Design review of the part shown in the three views and the two pictorial views. Dimensions are in mm from the part's minimum x, y and z. A direction names the side the tool comes from. Coordinates: 2 decimals unless noted, no trailing zeros. Loops run counter-clockwise (first coordinate to the right, second up) from the corner with the lowest first, then second, coordinate; pieces in that order, holes last.
Q1. Wall thickness on probe 1 along Z at (x, y) = (78.5, 21) (1 decimal); probe 2 along Y at (x, z) = (34, 14.25) (1 decimal); probe 3 along Z at (x, y) = (114, 1): over which ranges is each line inside the solid? List them lowest first.
Q2. Add section D-D on x = 115.5. Give the boundary of the cut face in (y, z) (1 decimal), and give its area (3 significant figures).
Q3. For P1, Ø7.5, axis at x = 114.3, z = 12.7, coming from the +Y side (3 decimals), flat-tipped, find the tip position at first contact; note if it passes through.
Q4. Machinability: for the marked faces 1 and 2, which of the approach directions +Z, -Z, +X, -X, +Y, -Y give a long, thin tool a straight path to every point of the face, cutting with its end or side? Answer none if there is none.
Q5. Add section B-B on x = 53. Give the boundary of the cut face in (y, z) (1 decimal).
Q6. Draft analysis for pull direction Z (two halves, no side actions). For the marked faces 3, 4, 5 and 6, state which applies: released by +Z, released by -Z, zero draft, split by the parting line, or undercut.
Q7. Add section C-C on y = 14.5. Give the boundary of the cut face in (x, z) (1 decimal).
Q8. Add section A-A on z = 12.7. Give the boundary of the cut face in (x, y) (1 decimal), and give its area (3 significant figures).
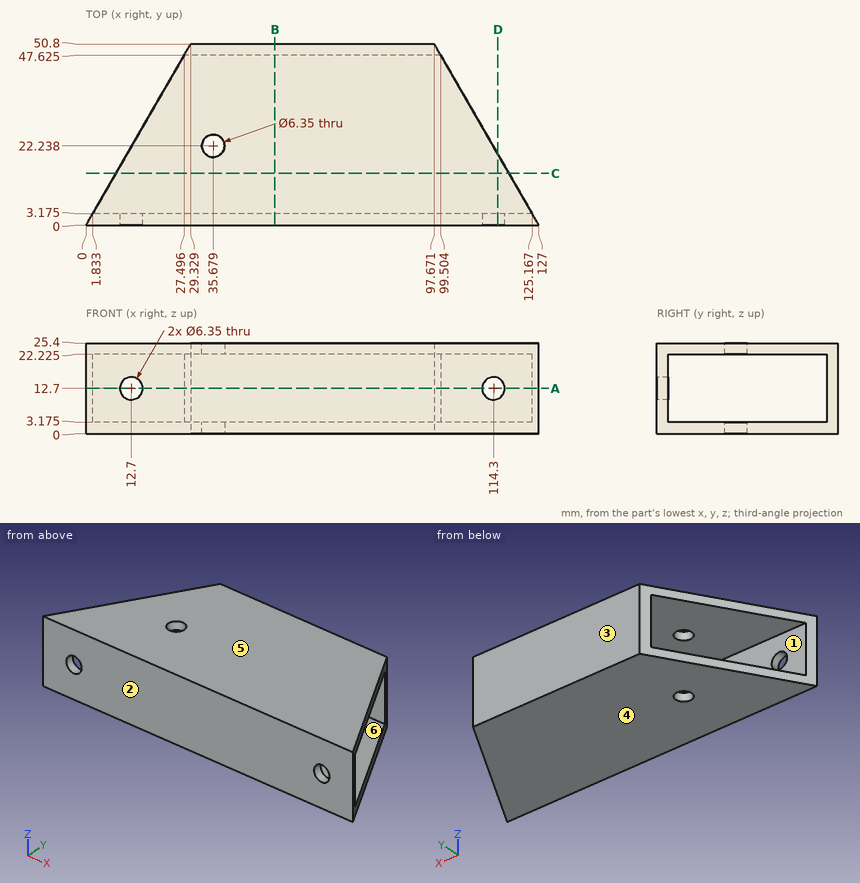
Entries:
1. probe 1: z = 0 to 3.2, 22.2 to 25.4
1. probe 2: y = 0 to 3.2, 47.6 to 50.8
1. probe 3: z = 0 to 9.54, 15.86 to 25.4
2. outline: (0, 0) - (19.9, 0) - (19.9, 3.2) - (3.2, 3.2) - (3.2, 9.8) - (0, 9.8) - close; (0, 15.6) - (3.2, 15.6) - (3.2, 22.2) - (19.9, 22.2) - (19.9, 25.4) - (0, 25.4) - close
2. area: 168 mm2
3. P1: stops at y = 3.175
4. face 1: +X, -X
4. face 2: +Z, -Z, +X, -X, -Y
5. outline: (0, 0) - (50.8, 0) - (50.8, 25.4) - (0, 25.4) - close; hole (3.2, 3.2) - (47.6, 3.2) - (47.6, 22.2) - (3.2, 22.2) - close
6. face 3: zero draft
6. face 4: released by -Z
6. face 5: released by +Z
6. face 6: undercut
7. outline: (8.4, 0) - (118.6, 0) - (118.6, 3.2) - (8.4, 3.2) - close; (8.4, 22.2) - (118.6, 22.2) - (118.6, 25.4) - (8.4, 25.4) - close
8. outline: (0, 0) - (9.5, 0) - (9.5, 3.2) - (1.8, 3.2) - close; (15.9, 0) - (111.1, 0) - (111.1, 3.2) - (15.9, 3.2) - close; (27.5, 47.6) - (99.5, 47.6) - (97.7, 50.8) - (29.3, 50.8) - close; (117.5, 0) - (127, 0) - (125.2, 3.2) - (117.5, 3.2) - close
8. area: 580 mm2
